Input: dimensioned drawing with shaded views. Units: mm. Origin: part minimum x, y, z. A direction names the side the tool comes from. Round coordinates to 2 decimals unless told otherwise and drop trailing zeros. Loops run counter-clockwise (first coordinate to the right, second up) from the corner with the lowest first, then second, coordinate; pieces in that order, holes last. Notation, with made-up numbers: (82, 51) - (111, 51) arc R21 cw to (111, 76) - close; hole circle Ø4 at (28, 15). An arc over 180 degrees is marked (long way). One line per question, with ' | ' between items.
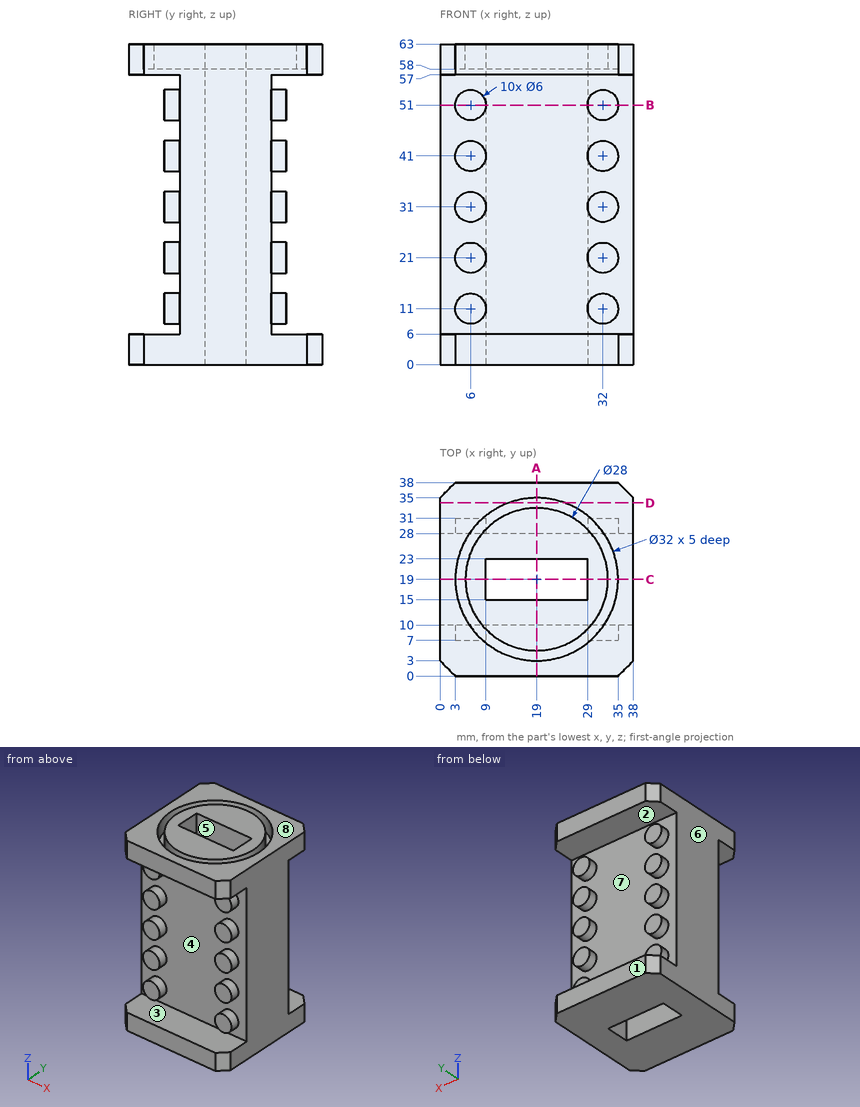
1. Mould query, pull axis Z, two halves, no side actions, for the marked faces 6, 7 and 8. Classes: released by +Z, released by -Z, zero draft, split by the parting line, or undercut.
Worked out:
face 6: zero draft | face 7: undercut | face 8: released by +Z
2. Access query for the marked faces 1, 2, 3, 4 and 5. Directions: +Z, -Z, +X, -X, +Y, -Y. A direction counts if a zero-diameter tool reaches every point of the face in a straight line with its end or side. Return the directions, or none.
Worked out:
face 1: +Z, -Z, +X, -X, +Y | face 2: +X, -X, +Y | face 3: +X, -X, -Y | face 4: -Y | face 5: +Z, -Z
3. Section query A-A, the plane x = 19. Return loops of the section in (y, z).
Worked out:
outline: (0, 0) - (15, 0) - (15, 63) - (5, 63) - (5, 58) - (3, 58) - (3, 63) - (0, 63) - (0, 57) - (10, 57) - (10, 6) - (0, 6) - close; (23, 0) - (38, 0) - (38, 6) - (28, 6) - (28, 57) - (38, 57) - (38, 63) - (35, 63) - (35, 58) - (33, 58) - (33, 63) - (23, 63) - close
4. Material intervals for probe 1 along Y at (x, z) = (19, 61.25); probe 2 along Y at (x, z) = (18, 48); probe 3 along Z at (x, y) = (2.5, 29.5), sorted ascending.
Worked out:
probe 1: y = 0 to 3, 5 to 15, 23 to 33, 35 to 38 | probe 2: y = 10 to 15, 23 to 28 | probe 3: z = 0 to 6, 57 to 63
5. Section query D-D, the plane y = 34. Return loops of the section in (x, z), plus the area to 3 significant figures.
Worked out:
outline: (0, 0) - (38, 0) - (38, 6) - (0, 6) - close; (0, 57) - (38, 57) - (38, 63) - (24.57, 63) - (24.57, 58) - (13.43, 58) - (13.43, 63) - (0, 63) - close | area: 400 mm2
6. Contact query for flat-ended pins moving along their axis: P1, Ø1.8, axis at x = 7, z = 11, coming from the -Y side; P2, Ø1.5, axis at x = 11, z = 38.5, coming from the -Y side; P3, Ø5, axis at x = 31.5, z = 31.5, coming from the +Y side. Output: stop coordinate, or through.
Worked out:
P1: stops at y = 7 | P2: stops at y = 10 | P3: stops at y = 31
7. Section query B-B, the plane z = 51. Return loops of the section in (x, y), plus the area to 3 significant figures.
Worked out:
outline: (0, 10) - (3, 10) - (3, 7) - (9, 7) - (9, 10) - (29, 10) - (29, 7) - (35, 7) - (35, 10) - (38, 10) - (38, 28) - (35, 28) - (35, 31) - (29, 31) - (29, 28) - (9, 28) - (9, 31) - (3, 31) - (3, 28) - (0, 28) - close; hole (9, 15) - (29, 15) - (29, 23) - (9, 23) - close | area: 596 mm2
8. Section query C-C, the plane y = 19. Return loops of the section in (x, z), plus the area to 3 significant figures.
Worked out:
outline: (0, 0) - (9, 0) - (9, 63) - (5, 63) - (5, 58) - (3, 58) - (3, 63) - (0, 63) - close; (29, 0) - (38, 0) - (38, 63) - (35, 63) - (35, 58) - (33, 58) - (33, 63) - (29, 63) - close | area: 1,110 mm2
